Here's how the part is built. I have some questions about the finished solid (model axes, mm). Face numbers are marked on the shaded views. A direction names the side the tool comes from. Coordinates: 2 decimals unless noted, no trailing zeros. Order: outer loops, then holes, each group sorted by start corner. A loop starts at its lowest first (then second) coordinate and runs counter-clockwise, first axis right, second up. Notation, with made-up numbers: (38, 74.25) - (91, 74.25) arc R20 ccw to (91, 113.25) - close; hole circle Ø6 at (52, -14.5). An arc over 180 degrees is marked (long way). Use one line per item in the form item = value. Start each with the question number.
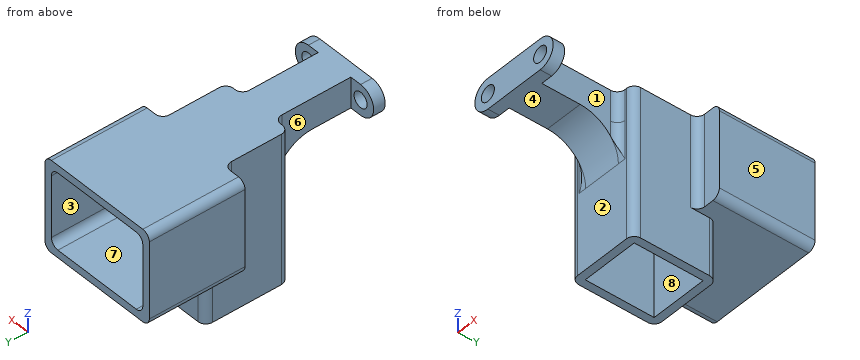
from build123d import *

# Parameters (mm, degrees)
SKETCH_1_R          = 2
EXTRUDE_1_DEPTH     = 3
SKETCH_2_W          = 10
SKETCH_2_H          = 8
EXTRUDE_2_DEPTH     = 20
SKETCH_3_W          = 19
SKETCH_3_H          = 39
EXTRUDE_3_DEPTH     = 22
SKETCH_4_W          = 15
SKETCH_4_H          = 18
CUT_EXTRUDE_1_DEPTH = 31
SKETCH_5_W          = 15
SKETCH_5_H          = 8
CUT_EXTRUDE_2_DEPTH = 5
SKETCH_6_W          = 32
SKETCH_6_H          = 24
EXTRUDE_5_DEPTH     = 20
SKETCH_7_W          = 28
SKETCH_7_H          = 20
CUT_EXTRUDE_3_DEPTH = 20
SKETCH_8_W          = 6.5
SKETCH_8_H          = 24
EXTRUDE_6_DEPTH     = 5
SKETCH_9_W          = 15
SKETCH_9_H          = 10
EXTRUDE_7_DEPTH     = 2
FILLET_1_R          = 2
FILLET_2_R          = 2
FILLET_3_R          = 2
FILLET_4_R          = 2
FILLET_5_R          = 2
FILLET_6_R          = 2
FILLET_7_R          = 2
FILLET_8_R          = 2
FILLET_9_R          = 2
FILLET_10_R         = 2
FILLET_11_R         = 2
FILLET_12_R         = 2
FILLET_13_R         = 2
FILLET_14_R         = 2
FILLET_15_R         = 2
FILLET_16_R         = 2
FILLET_17_R         = 2
FILLET_18_R         = 2
FILLET_19_R         = 2
FILLET_20_R         = 2
FILLET_START        = -5
FILLET_21_DEPTH     = 10
FILLET_START_2      = -14
FILLET_21_2_DEPTH   = 10
FILLET_START_3      = -8
FILLET_21_3_DEPTH   = 16


with BuildPart() as part:
    # 草图1 → 凸台-拉伸1 (new body)
    with BuildSketch(Plane(origin=(0, 0, 0), x_dir=(1, 0, 0), z_dir=(0, 1, 0))):
        with BuildLine():
            Line((-8, 4), (8, 4))
            ThreePointArc((8, 4), (12, 0), (8, -4))
            Line((8, -4), (-8, -4))
            ThreePointArc((-8, -4), (-12, 0), (-8, 4))
        make_face()
        with Locations(Location((8, 0, 0), (0, 0, 270))):
            Circle(SKETCH_1_R, mode=Mode.SUBTRACT)
        with Locations(Location((-8, 0, 0), (0, 0, 270))):
            Circle(SKETCH_1_R, mode=Mode.SUBTRACT)
    extrude(amount=EXTRUDE_1_DEPTH)

    # 草图2 → 凸台-拉伸2 (add)
    with BuildSketch(Plane(origin=(0, 3, 0), x_dir=(1, 0, 0), z_dir=(0, 1, 0))):
        Rectangle(SKETCH_2_W, SKETCH_2_H)
    extrude(amount=EXTRUDE_2_DEPTH)

    # 草图3 → 凸台-拉伸3 (add)
    with BuildSketch(Plane(origin=(0, 23, 0), x_dir=(1, 0, 0), z_dir=(0, 1, 0))):
        with Locations((0, 15.5)):
            Rectangle(SKETCH_3_W, SKETCH_3_H)
    extrude(amount=EXTRUDE_3_DEPTH)

    # 草图4 → 切除-拉伸1 (cut)
    with BuildSketch(Plane(origin=(0, 0, -35), x_dir=(-1, 0, 0), z_dir=(0, 0, -1))):
        with Locations((0, 34)):
            Rectangle(SKETCH_4_W, SKETCH_4_H)
    extrude(amount=-CUT_EXTRUDE_1_DEPTH, mode=Mode.SUBTRACT)

    # 草图5 → 切除-拉伸2 (cut)
    with BuildSketch(Plane(origin=(0, 45, 0), x_dir=(1, 0, 0), z_dir=(0, 1, 0))):
        with Locations((0, 8)):
            Rectangle(SKETCH_5_W, SKETCH_5_H)
    extrude(amount=-CUT_EXTRUDE_2_DEPTH, mode=Mode.SUBTRACT)

    # 草图6 → 凸台-拉伸5 (add)
    with BuildSketch(Plane(origin=(0, 45, 0), x_dir=(1, 0, 0), z_dir=(0, 1, 0))):
        with Locations((0, 8)):
            Rectangle(SKETCH_6_W, SKETCH_6_H)
    extrude(amount=EXTRUDE_5_DEPTH)

    # 草图7 → 切除-拉伸3 (cut)
    with BuildSketch(Plane(origin=(0, 65, 0), x_dir=(1, 0, 0), z_dir=(0, 1, 0))):
        with Locations((0, 8)):
            Rectangle(SKETCH_7_W, SKETCH_7_H)
    extrude(amount=-CUT_EXTRUDE_3_DEPTH, mode=Mode.SUBTRACT)

    # 草图8 → 凸台-拉伸6 (add)
    with BuildSketch(Plane(origin=(0, 45, 0), x_dir=(1, 0, 0), z_dir=(0, 1, 0))):
        Polygon((-16, 20), (-16, -4), (-9.5, -4), (-9.5, -2), (-9.5, 18), (-9.5, 20), align=None)
        with Locations((12.75, 8)):
            Rectangle(SKETCH_8_W, SKETCH_8_H)
    extrude(amount=-EXTRUDE_6_DEPTH)

    # 草图9 → 凸台-拉伸7 (add)
    with BuildSketch(Plane(origin=(0, 25, 0), x_dir=(1, 0, 0), z_dir=(0, 1, 0))):
        with Locations((0, 9)):
            Rectangle(SKETCH_9_W, SKETCH_9_H)
    extrude(amount=EXTRUDE_7_DEPTH)

    # 圆角1
    fillet_1_edges = [part.edges().sort_by_distance(p)[0] for p in [
        (16, 52.5, -20),
    ]]
    fillet(fillet_1_edges, radius=FILLET_1_R)

    # 圆角2
    fillet_2_edges = [part.edges().sort_by_distance(p)[0] for p in [
        (-16, 52.5, -20),
    ]]
    fillet(fillet_2_edges, radius=FILLET_2_R)

    # 圆角3
    fillet_3_edges = [part.edges().sort_by_distance(p)[0] for p in [
        (-16, 52.5, 4),
    ]]
    fillet(fillet_3_edges, radius=FILLET_3_R)

    # 圆角4
    fillet_4_edges = [part.edges().sort_by_distance(p)[0] for p in [
        (16, 52.5, 4),
    ]]
    fillet(fillet_4_edges, radius=FILLET_4_R)

    # 圆角5
    fillet_5_edges = [part.edges().sort_by_distance(p)[0] for p in [
        (14, 55, 2),
    ]]
    fillet(fillet_5_edges, radius=FILLET_5_R)

    # 圆角6
    fillet_6_edges = [part.edges().sort_by_distance(p)[0] for p in [
        (-14, 55, 2),
    ]]
    fillet(fillet_6_edges, radius=FILLET_6_R)

    # 圆角7
    fillet_7_edges = [part.edges().sort_by_distance(p)[0] for p in [
        (-14, 55, -18),
    ]]
    fillet(fillet_7_edges, radius=FILLET_7_R)

    # 圆角8
    fillet_8_edges = [part.edges().sort_by_distance(p)[0] for p in [
        (14, 55, -18),
    ]]
    fillet(fillet_8_edges, radius=FILLET_8_R)

    # 圆角9
    fillet_9_edges = [part.edges().sort_by_distance(p)[0] for p in [
        (-7.5, 36, -4),
    ]]
    fillet(fillet_9_edges, radius=FILLET_9_R)

    # 圆角10
    fillet_10_edges = [part.edges().sort_by_distance(p)[0] for p in [
        (7.5, 36, -4),
    ]]
    fillet(fillet_10_edges, radius=FILLET_10_R)

    # 圆角11
    fillet_11_edges = [part.edges().sort_by_distance(p)[0] for p in [
        (7.5, 44, -12),
    ]]
    fillet(fillet_11_edges, radius=FILLET_11_R)

    # 圆角12
    fillet_12_edges = [part.edges().sort_by_distance(p)[0] for p in [
        (-7.5, 44, -12),
    ]]
    fillet(fillet_12_edges, radius=FILLET_12_R)

    # 圆角13
    fillet_13_edges = [part.edges().sort_by_distance(p)[0] for p in [
        (-9.5, 45, -27.5),
    ]]
    fillet(fillet_13_edges, radius=FILLET_13_R)

    # 圆角14
    fillet_14_edges = [part.edges().sort_by_distance(p)[0] for p in [
        (9.5, 45, -27.5),
    ]]
    fillet(fillet_14_edges, radius=FILLET_14_R)

    # 圆角15
    fillet_15_edges = [part.edges().sort_by_distance(p)[0] for p in [
        (9.5, 23, -15.5),
    ]]
    fillet(fillet_15_edges, radius=FILLET_15_R)

    # 圆角16
    fillet_16_edges = [part.edges().sort_by_distance(p)[0] for p in [
        (-9.5, 23, -15.5),
    ]]
    fillet(fillet_16_edges, radius=FILLET_16_R)

    # 圆角17
    fillet_17_edges = [part.edges().sort_by_distance(p)[0] for p in [
        (9.5, 40, -8),
    ]]
    fillet(fillet_17_edges, radius=FILLET_17_R)

    # 圆角18
    fillet_18_edges = [part.edges().sort_by_distance(p)[0] for p in [
        (-9.5, 40, -8),
    ]]
    fillet(fillet_18_edges, radius=FILLET_18_R)

    # 圆角19
    fillet_19_edges = [part.edges().sort_by_distance(p)[0] for p in [
        (5, 23, 0),
    ]]
    fillet(fillet_19_edges, radius=FILLET_19_R)

    # 圆角20
    fillet_20_edges = [part.edges().sort_by_distance(p)[0] for p in [
        (-5, 23, 0),
    ]]
    fillet(fillet_20_edges, radius=FILLET_20_R)

    # 圆角21: read off the stored shape, not the designer's step
    # 圆角21 outline → 圆角21 (add)
    with BuildSketch(Plane.YZ.offset(FILLET_START)):
        with BuildLine():
            Line((23, -4), (13, -4))
            ThreePointArc((13, -4), (20.071068, -6.928932), (23, -14))
            Line((23, -14), (23, -4))
        make_face()
    extrude(amount=FILLET_21_DEPTH)

    # Fillet 21 2 outline → Fillet 21 2 (add)
    with BuildSketch(Plane.XY.offset(FILLET_START_2)):
        with BuildLine():
            Line((5, 23), (5, 21))
            ThreePointArc((5, 21), (5.585786, 22.414214), (7, 23))
            Line((7, 23), (5, 23))
        make_face()
        with BuildLine():
            Line((-5, 21), (-5, 23))
            Line((-5, 23), (-7, 23))
            ThreePointArc((-7, 23), (-5.585786, 22.414214), (-5, 21))
        make_face()
    extrude(amount=FILLET_21_2_DEPTH)

    # Fillet 21 3 outline → Fillet 21 3 (cut)
    with BuildSketch(Plane.YZ.offset(FILLET_START_3)):
        with BuildLine():
            Line((21, -14), (23, -14))
            ThreePointArc((23, -14), (22.486833, -10.837722), (21, -8))
            Line((21, -8), (21, -14))
        make_face()
    extrude(amount=FILLET_21_3_DEPTH, mode=Mode.SUBTRACT)


solid = part.part
1) Suppose I cut it at C-C, the plane y = 18. List the corners of the cut face in (x, z) for me.
2) If we mould it in two halves opening along X, with no side actions, what happens to the marked faces 1, 2 and 3? For each: pulls with the +X half, pulls with the -X half, needs draft (parallel to the pull), parting line crosses it, or undercut.
3) Which directions (+Z, -Z, +X, -X, +Y, -Y) give clear straight access to the entire face, cutting with the end or side of a thin tool? Please do the marked faces 4, 5, 6, 7 and 8.
4) Suppose I cut it at A-A, the plane x = 1.5. List the corners of the cut face in (y, z) for me.
5) Suppose I cut it at B-B, the plane z = -31. List the corners of the cut face in (x, y) for me, then the cut area to 3 significant figures.
6) For pin 1 (4 mm diameter, centred on x = 0.5, y = 3.5, fed in from -Z); pin 2 (5.5 mm diameter, centred on x = 8, z = -1.5, fed in from +Y); pin 3 (2 mm diameter, centred on x = 5, z = -11.5, fed in from -Y); pin 4 (22 mm diameter, centred on y = 34, z = -17.5, fed in from +X), each with a flat end and sliding along its axis, tell me the tip position at first contact or that it passes through.
7) I need wall thicknesses on probe 1 along X at (y, z) = (2, 0); probe 2 along Y at (x, z) = (-4.5, -23.5); probe 3 along Z at (x, y) = (11, 61.5). Which ranges of each line are inside material? Lowest first, please. Write a range as [from, to].
From the geometry:
q1.outline = (-5, -5.34) - (5, -5.34) - (5, 4) - (-5, 4) - close
q2.face_1 = pulls with the +X half
q2.face_2 = needs draft
q2.face_3 = undercut
q3.face_4 = -Z, +X, -X, -Y
q3.face_5 = +Z, -Z, +X, +Y, -Y
q3.face_6 = +Z, -Z, -X
q3.face_7 = +Y
q3.face_8 = -Z
q4.outline = (0, -4) - (13, -4) arc R10 cw to (23, -14) - (23, -35) - (25, -35) - (25, -14) - (27, -14) - (27, -4) - (45, -4) - (45, 2) - (65, 2) - (65, 4) - (0, 4) - close; (43, -35) - (45, -35) - (45, -20) - (65, -20) - (65, -18) - (45, -18) - (45, -12) - (43, -12) - close
q5.outline = (-9.5, 25) arc R2 ccw to (-7.5, 23) - (7.5, 23) arc R2 ccw to (9.5, 25) - (9.5, 43) arc R2 ccw to (7.5, 45) - (-7.5, 45) arc R2 ccw to (-9.5, 43) - close; hole (-7.5, 25) - (7.5, 25) - (7.5, 43) - (-7.5, 43) - close
q5.area = 145 mm2
q6.pin_1 = -4
q6.pin_2 = 45
q6.pin_3 = 22.37
q6.pin_4 = 16
q7.probe_1 = [-12, -10], [-6, 6], [10, 12]
q7.probe_2 = [23, 25], [43, 45]
q7.probe_3 = [-20, -18], [2, 4]
